from build123d import *

# Parameters (mm, degrees)
FRONT_PROFILE_W           = 31.75
FRONT_PROFILE_H           = 25.4
FRONT_PROFILE_R           = 4
WEPON_MOTOR_MOINT_DEPTH   = 6.35
F_3_0MM_DOWEL_HOLE1_D     = 3
CIRPATTERN1_COUNT         = 4
F_3_0MM_DOWEL_HOLE2_D     = 3
F_3_0MM_DOWEL_HOLE2_DEPTH = 5
F_3_0MM_DOWEL_HOLE2_TIP   = 0.901290929


with BuildPart() as part:
    # front profile → wepon motor moint (new body)
    with BuildSketch(Plane.XY):
        with Locations((-15.875, 12.7)):
            Rectangle(FRONT_PROFILE_W, FRONT_PROFILE_H)
        with Locations((-15.875, 10.4)):
            Circle(FRONT_PROFILE_R, mode=Mode.SUBTRACT)
    extrude(amount=WEPON_MOTOR_MOINT_DEPTH)

    # Ø3.0mm Dowel Hole1 (through all)
    with Locations(Plane.XY.offset(6.35)):
        with Locations((-21.531854249, 16.056854249)):
            f_3_0mm_dowel_hole1 = Hole(F_3_0MM_DOWEL_HOLE1_D / 2)

    # CirPattern1: Ø3.0mm Dowel Hole1 ×4 about axis
    cirpattern1_axis = Axis((-15.875, 10.4, 0), (0, 0, 1))
    for i in range(1, CIRPATTERN1_COUNT):
        add(f_3_0mm_dowel_hole1.rotate(cirpattern1_axis, i * 360 / CIRPATTERN1_COUNT), mode=Mode.SUBTRACT)

    # Ø3.0mm Dowel Hole2
    with Locations(Plane(origin=(0, 0, 0), x_dir=(-1, 0, 0), z_dir=(0, -1, 0))):
        with Locations((6.35, -3.175), (25.4, -3.175)):
            Hole(F_3_0MM_DOWEL_HOLE2_D / 2, depth=F_3_0MM_DOWEL_HOLE2_DEPTH)
            with Locations((0, 0, -(F_3_0MM_DOWEL_HOLE2_DEPTH + F_3_0MM_DOWEL_HOLE2_TIP / 2))):  # 118° drill point
                Cone(0, F_3_0MM_DOWEL_HOLE2_D / 2, F_3_0MM_DOWEL_HOLE2_TIP, mode=Mode.SUBTRACT)


solid = part.part
The listing builds one solid part. Answer for the finished solid, in the listing's coordinates (mm). A direction names the side the tool comes from. Round coordinates to 2 decimals unless told otherwise and drop trailing zeros. Loops run counter-clockwise (first coordinate to the right, second up) from the corner with the lowest first, then second, coordinate; pieces in that order, holes last. Notation, with made-up numbers: M 42,37 L 78,37 A28 cw 78,73 Z; hole C -14.5,30 d7. An arc over 180 degrees is marked long. Return JSON: item names as keys, results as strings.
Q1. Find the intervals of material crossed by line 1 along Y through (x, z) = (-21.5, 4.5); line 2 along Y through (x, z) = (-11, 6); line 3 along Z through (x, y) = (-25.4, 3.45) (3 decimals), in increasing order. Write a range as from..to.
Results list:
{"line 1": "y = 0..3.24, 6.24..14.56, 17.56..25.4", "line 2": "y = 0..3.46, 6.02..14.78, 17.34..25.4", "line 3": "z = 0..1.675, 4.675..6.35"}
Q2. Find section B-B, the plane x = -16. Determine the outline of the cut face in (y, z), plus the area to 3 significant figures.
Results list:
{"outline": "M 0,0 L 6.4,0 L 6.4,6.35 L 0,6.35 Z; M 14.4,0 L 25.4,0 L 25.4,6.35 L 14.4,6.35 Z", "area": "111 mm2"}
Q3. Find section D-D, the plane z = 0.5. Determine the outline of the cut face in (x, y) (3 decimals).
Results list:
{"outline": "M -31.75,0 L 0,0 L 0,25.4 L -31.75,25.4 Z; hole C -21.532,4.743 d3; hole C -21.532,16.057 d3; hole C -15.875,10.4 d8; hole C -10.218,4.743 d3; hole C -10.218,16.057 d3"}
Q4. The mould has two halves that part along Y. Classify faces 3 (the face through (-16, 0, 3)), 4 (the face through (-16, 16, 6.35)), 5 (the face through (-19.87, 10.58, 3.13)), 6 (the face through (-11.131, 14.867, 3.131)): released by +Y, released by -Y, zero draft, split by the parting line, or undercut.
Results list:
{"face 3": "released by -Y", "face 4": "zero draft", "face 5": "undercut", "face 6": "undercut"}
Q5. Find section A-A, the plane y = 10.4. Determine the outline of the cut face in (x, z) (3 decimals), plus the area to 3 significant figures.
Results list:
{"outline": "M -31.75,0 L -19.875,0 L -19.875,6.35 L -31.75,6.35 Z; M -11.875,0 L 0,0 L 0,6.35 L -11.875,6.35 Z", "area": "151 mm2"}
Q6. Which of the six approach directions +Z, -Z, +X, -X, +Y, -Y give full straight-line access (tool end or side, diameter ignored) to faces 1 (the face through (-26.9, 2.5, 3.1)), 2 (the face through (-31.75, 13, 3))?
Results list:
{"face 1": "-Y", "face 2": "+Z, -Z, -X, +Y, -Y"}
Q7. Find section C-C, the plane x = -22.5. Determine the outline of the cut face in (y, z).
Results list:
{"outline": "M 0,0 L 3.6,0 L 3.6,6.35 L 0,6.35 Z; M 5.89,0 L 14.91,0 L 14.91,6.35 L 5.89,6.35 Z; M 17.2,0 L 25.4,0 L 25.4,6.35 L 17.2,6.35 Z"}
